CAD build for the part. Positions are in the model's coordinates, mm. A direction names the side the tool comes from. Round coordinates to 2 decimals unless told otherwise and drop trailing zeros.
```python
from build123d import *

# Parameters (mm, degrees)
F0_W     = 104.1534732964
F0_H     = 76.8153294921
F4_R     = 29.4148902483
F5_DEPTH = 127


# Not quite as in the source:
# - the arcs of a loft's sections are written as splines that run evenly, so that the points pair up as in the source's solid


with BuildPart() as f3:
    # F0 (on Top) → F3 section 0
    with BuildSketch(Plane.XY):
        with Locations((12.8655565871, 0)):
            Rectangle(F0_W, F0_H)
    # F2 (on offset) → F3 section 1
    with BuildSketch(Plane.XY.offset(152.4)):
        with BuildLine():
            add(Edge.make_bspline(
                [(-41.6450555416, 40.7195541248), (-43.8796016064, 38.3671029534), (-45.8824019296, 35.7946318153), (-49.3477407941, 30.3082562291), (-50.810193648, 27.3944874425), (-53.1386082181, 21.3374769498), (-54.0045123596, 18.1943850152), (-55.1065229691, 11.7995071325), (-55.3426021877, 8.5478793103), (-55.175859187, 2.0608856083), (-54.7730410907, -1.1743198678), (-53.3439523197, -7.5041378591), (-52.3177169821, -10.5985938571), (-49.6812015209, -16.5279847821), (-48.0709865904, -19.3627730932), (-44.3283642496, -24.6638737839), (-42.196049383, -27.1300550832), (-39.8435982116, -29.3646011481)],
                knots=[0, 0, 0, 0, 0.125, 0.125, 0.25, 0.25, 0.375, 0.375, 0.5, 0.5, 0.625, 0.625, 0.75, 0.75, 0.875, 0.875, 1, 1, 1, 1], degree=3))
            add(Edge.make_bspline(
                [(-39.8435982116, -29.3646011481), (-37.4911470402, -31.5991472129), (-34.9186759021, -33.6019475362), (-29.4323003159, -37.0672864006), (-26.5185315293, -38.5297392545), (-20.4615210366, -40.8581538246), (-17.318429102, -41.7240579661), (-10.9235512193, -42.8260685756), (-7.6719233971, -43.0621477942), (-1.1849296951, -42.8954047935), (2.050275781, -42.4925866972), (8.3800937724, -41.0634979262), (11.4745497703, -40.0372625886), (17.4039406953, -37.4007471274), (20.2387290065, -35.7905321969), (25.5398296971, -32.0479098561), (28.0060109965, -29.9155949895), (30.2405570613, -27.5631438181)],
                knots=[0, 0, 0, 0, 0.125, 0.125, 0.25, 0.25, 0.375, 0.375, 0.5, 0.5, 0.625, 0.625, 0.75, 0.75, 0.875, 0.875, 1, 1, 1, 1], degree=3))
            add(Edge.make_bspline(
                [(30.2405570613, -27.5631438181), (32.4751031261, -25.2106926468), (34.4779034494, -22.6382215086), (37.9432423138, -17.1518459224), (39.4056951677, -14.2380771358), (41.7341097378, -8.1810666431), (42.6000138793, -5.0379747085), (43.7020244888, 1.3569031742), (43.9381037074, 4.6085309964), (43.7713607067, 11.0955246984), (43.3685426104, 14.3307301745), (41.9394538394, 20.6605481658), (40.9132185018, 23.7550041638), (38.2767030406, 29.6843950888), (36.6664881101, 32.5191833999), (32.9238657693, 37.8202840906), (30.7915509027, 40.2864653899), (28.4390997313, 42.5210114548)],
                knots=[0, 0, 0, 0, 0.125, 0.125, 0.25, 0.25, 0.375, 0.375, 0.5, 0.5, 0.625, 0.625, 0.75, 0.75, 0.875, 0.875, 1, 1, 1, 1], degree=3))
            add(Edge.make_bspline(
                [(28.4390997313, 42.5210114548), (26.08664856, 44.7555575196), (23.5141774218, 46.7583578429), (18.0278018356, 50.2236967073), (15.114033049, 51.6861495612), (9.0570225563, 54.0145641313), (5.9139306218, 54.8804682728), (-0.480947261, 55.9824788823), (-3.7325750832, 56.2185581009), (-10.2195687852, 56.0518151002), (-13.4547742613, 55.6489970039), (-19.7845922526, 54.2199082329), (-22.8790482506, 53.1936728953), (-28.8084391756, 50.5571574341), (-31.6432274867, 48.9469425036), (-36.9443281774, 45.2043201628), (-39.4105094767, 43.0720052962), (-41.6450555416, 40.7195541248)],
                knots=[0, 0, 0, 0, 0.125, 0.125, 0.25, 0.25, 0.375, 0.375, 0.5, 0.5, 0.625, 0.625, 0.75, 0.75, 0.875, 0.875, 1, 1, 1, 1], degree=3))
        make_face()
    loft(ruled=True)

    # F4 (on face) → F5 (cut)
    with BuildSketch(Plane.XY.offset(152.4)):
        with Locations((0, 5.3224205039)):
            Circle(F4_R)
    extrude(amount=-F5_DEPTH, mode=Mode.SUBTRACT)


solid = f3.part
```
Item 1: Flat gauge pins, fed straight in: P1, Ø10, axis at y = 37, z = 122, coming from the +X side; P2, Ø3, axis at x = 23, z = 41.5, coming from the -Y side; P3, Ø3, axis at x = -3, y = -21.5, coming from the +Z side. Where does each tip first touch, or does it go through?
Answers follow:
P1: stops at x = 41.93
P2: stops at y = -39.26
P3: stops at z = 25.4
Item 2: 3-axis set-ups, long thin cutter, end or side, ignore diameter. For faces 3 (the cylindrical face through (-3.829, 34.487, 89.789)), 4 (the flat face through (12, 0, 0)): which of +Z, -Z, +X, -X, +Y, -Y reach the whole face in a straight line?
Answers follow:
face 3: +Z
face 4: -Z, +X, -X, +Y, -Y
Item 3: Probe line 1 (Z direction, x = 15, y = -11); line 2 (Y direction, x = -7, z = 33); line 3 (Y direction, x = 23, z = 91.5). List the from-to ranges inside material, lowest first.
Answers follow:
line 1: z = 0 to 25.4
line 2: y = -39.11 to -23.25, 33.89 to 41.85
line 3: y = -38.86 to -13.01, 23.66 to 47.04
Item 4: Two-plate mould, pull along X, no slides. Class faces 1 (the flat face through (-29, -1, 152.4)), 2 (the flat face through (0, 6, 25.4)): released by +X, released by -X, zero draft, split by the parting line, or undercut.
Answers follow:
face 1: zero draft
face 2: undercut
